Part model, mm, in its own coordinate system. Round coordinates to 2 decimals unless told otherwise and drop trailing zeros. Write each loop counter-clockwise with the first axis right and the second up, starting at its lowest first coordinate (ties: lowest second). Pieces come first, ordered by that corner, then holes.
```python
from build123d import *

# Parameters (mm, degrees)
BOX_W             = 160
BOX_H             = 100
BOX_DEPTH         = 3
BOX001_W          = 126
BOX001_H          = 76
BOX001_DEPTH      = 5
BOX023_W          = 153.6
BOX023_H          = 3
BOX023_DEPTH      = 4
BOX024_W          = 3.8
BOX024_H          = 3.8
BOX024_DEPTH      = 4.6
CYLINDER012_R     = 1.9
CYLINDER012_DEPTH = 8.6
FILLET_R          = 10
FILLET015_R       = 5
PAD021_DEPTH      = 76.8


with BuildPart() as part:
    # Box → Box (join)
    with BuildSketch(Plane(origin=(-80, -50, -5), x_dir=(1, 0, 0), z_dir=(0, 0, 1))):
        with Locations((80, 50)):
            Rectangle(BOX_W, BOX_H)
    extrude(amount=BOX_DEPTH)

    # Box001 → Box001 (cut)
    with BuildSketch(Plane(origin=(-63, -38, -6), x_dir=(1, 0, 0), z_dir=(0, 0, 1))):
        with Locations((63, 38)):
            Rectangle(BOX001_W, BOX001_H)
    extrude(amount=BOX001_DEPTH, mode=Mode.SUBTRACT)

    # Box023 → Box023 (join)
    with BuildSketch(Plane(origin=(-76.8, 43.8, -9), x_dir=(1, 0, 0), z_dir=(0, 0, 1))):
        with Locations((76.8, 1.5)):
            Rectangle(BOX023_W, BOX023_H)
    extrude(amount=BOX023_DEPTH)

    # Box024 → Box024 (join)
    with BuildSketch(Plane(origin=(68.6, -41.9, -9.6), x_dir=(1, 0, 0), z_dir=(0, 0, 1))):
        with Locations((1.9, 1.9)):
            Rectangle(BOX024_W, BOX024_H)
    box024 = extrude(amount=BOX024_DEPTH)

    # Cylinder012 → Cylinder012 (join)
    with BuildSketch(Plane(origin=(66.2, -40, -9.6), x_dir=(0, 1, 0), z_dir=(1, 0, 0))):
        Circle(CYLINDER012_R)
    cylinder012 = extrude(amount=CYLINDER012_DEPTH)

    # Mirrored006: Box024, Cylinder012 across YZ
    add(box024.mirror(Plane.YZ))
    add(cylinder012.mirror(Plane.YZ))

    # Fillet
    fillet_edges = [part.edges().sort_by_distance(p)[0] for p in [
        (80, -50, -3.5),
    ]]
    fillet(fillet_edges, radius=FILLET_R)

    # Fillet015
    fillet015_edges = [part.edges().sort_by_distance(p)[0] for p in [
        (-80, -50, -3.5),
    ]]
    fillet(fillet015_edges, radius=FILLET015_R)

    # Sketch038 → Pad021 (join, symmetric)
    with BuildSketch(Plane.YZ):
        Polygon((46.8, -6.653981), (46.8, -8.5), (47.9, -7.57699), align=None)
    extrude(amount=PAD021_DEPTH, both=True)


solid = part.part
```
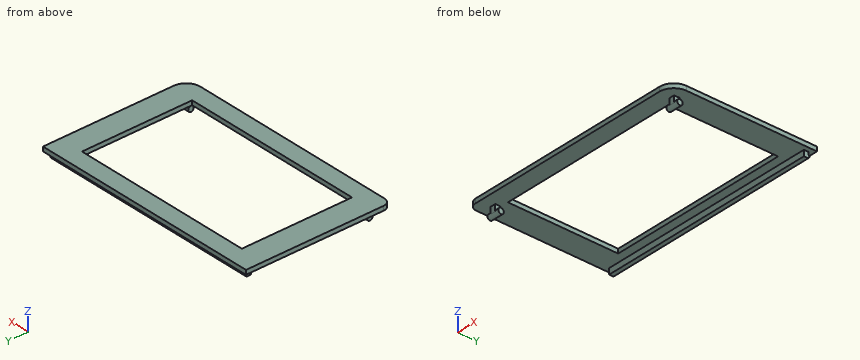
Q1. Drop flat-ended pins along their axis: pin 1 (1 mm diameter, centred on x = -34, z = -8.5, fed in from +Y); pin 2 (3 mm diameter, centred on y = -40.5, z = -7.5, fed in from -X); pin 3 (1.1 mm diameter, centred on x = -70, z = -7.5, fed in from +Y). Give the stop position or say it passes through.
Values follow:
pin 1: stops at y = 47.4
pin 2: stops at x = -74.8
pin 3: stops at y = 47.9
Q2. Cut at A-A on x = 44. Write the cut outline in (y, z), plus the area to 3 significant figures.
Values follow:
outline: (-50, -5) - (-38, -5) - (-38, -2) - (-50, -2) - close; (38, -5) - (43.8, -5) - (43.8, -9) - (46.8, -9) - (46.8, -8.5) - (47.9, -7.58) - (46.8, -6.65) - (46.8, -5) - (50, -5) - (50, -2) - (38, -2) - close
area: 85.0 mm2
Q3. Wall check: L1, parallel to Z at x = 65, y = -20.5; L2, parallel to Y at x = 39.5, z = -3; L3, parallel to Z at x = 44, y = 45. Give the ranges that are in metal, low to high.
Values follow:
L1: z = -5 to -2
L2: y = -50 to -38, 38 to 50
L3: z = -9 to -2
Q4. Cut at B-B on y = -29. Write the cut outline in (x, z), plus the area to 3 significant figures.
Values follow:
outline: (-80, -5) - (-63, -5) - (-63, -2) - (-80, -2) - close; (63, -5) - (80, -5) - (80, -2) - (63, -2) - close
area: 102 mm2
